```python
from build123d import *

# Parameters (mm, degrees)
F1_DEPTH = 6
F2_R     = 2.5
F3_DEPTH = 50


with BuildPart() as f1:
    # F0 (on Top) → F1 (new body)
    with BuildSketch(Plane.XY):
        Polygon((5, -10), (10, -10), (10, -2), (15, -2), (15, 10), (11, 10), (11, 2), (-11, 2), (-11, 10), (-15, 10), (-15, -2), (-10, -2), (-10, -10), (-5, -10), (-5, -2), (5, -2), align=None)
    extrude(amount=F1_DEPTH)

    # F2 (on face) → F3 (cut)
    with BuildSketch(Plane(origin=(-15, 0, 0), x_dir=(0, -1, 0), z_dir=(-1, 0, 0))):
        with Locations((-6.949849, 3)):
            Circle(F2_R)
        with BuildLine():
            ThreePointArc((-6.949849, 0), (-9.949849, 3), (-6.949849, 6))
            Line((-6.949849, 6), (-10, 6))
            Line((-10, 6), (-10, 0))
            Line((-10, 0), (-6.949849, 0))
        make_face()
        with Locations((6.964043, 3)):
            Circle(F2_R)
        with BuildLine():
            Line((10, 6), (6.964043, 6))
            ThreePointArc((6.964043, 6), (9.085363, 5.12132), (9.964043, 3))
            ThreePointArc((9.964043, 3), (9.085363, 0.87868), (6.964043, 0))
            Line((6.964043, 0), (10, 0))
            Line((10, 0), (10, 6))
        make_face()
    extrude(amount=-F3_DEPTH, mode=Mode.SUBTRACT)


solid = f1.part
```
Build history of the part. All positions in model axes, mm. A direction names the side the tool comes from. Coordinates: 2 decimals unless noted, no trailing zeros. Order: outer loops, then holes, each group sorted by start corner. A loop starts at its lowest first (then second) coordinate and runs counter-clockwise, first axis right, second up. Notation, with made-up numbers: (87, 18.25) -> (127, 18.25) arc R12 ccw to (127, 32.25) -> close; hole circle Ø4 at (81, 49.5). An arc over 180 degrees is marked (long way). Answer in a Markdown table with one row per item. Add a question column.
Q1. Which spindle directions (+Z, -Z, +X, -X, +Y, -Y) get a long thin tool onto all of the face, cutting with end or side? Do faces 4 (the face through (-13, -2, 3)), 5 (the face through (0, 2, 3)), 6 (the face through (12, -2, 3)), 7 (the face through (0, -2, 3)). Say none if no direction does.
Q2. Drop flat-ended pins along their axis: pin 1 (1.5 mm diameter, centred on x = -6, z = 4.5, fed in from -Y); pin 2 (3 mm diameter, centred on y = -6.96, z = 3, fed in from -X); pin 3 (3 mm diameter, centred on x = -9, z = 4, fed in from +Y); pin 4 (1.8 mm diameter, centred on y = -4.5, z = 2.5, fed in from -X). Give the stop position or say it passes through.
Q3. Mould opens along Y. For faces 1 (the face through (12.97, 9.95, 2.93)), 2 (the face through (0, 0, 0)), 3 (the face through (-13.028, 9.447, 3.11)) say: +Y half, -Y half, draft (parallel to the pull), parting line (faces both ways), or undercut.
Q4. Band-saw the part on D-D, the plane z = 4. Give the number of separate pieces and of enclosed holes in the cut face, then the cut area to 3 significant figures.
Q5. Wall check: line 1 along X through (y, z) = (-3.5, 5); line 2 along X through (y, z) = (2.75, 5.5); line 3 along Y through (x, z) = (12.5, 1.25). Give the ranges that are in metal, low to high. Write a range as [from, to].
Q6. Band-saw the part on C-C, the plane y = -8.75. List the corners of the cut face in (x, z), then the cut area to 3 significant figures.
Q7. Band-saw the part on A-A, the plane y = -4. List the corners of the cut face in (x, z), then the cut area to 3 significant figures.
Q8. Band-saw the part on B-B, the plane x = 9.5. List the corners of the cut face in (y, z).
Answers follow:
| question | item | result |
|---|---|---|
| 1 | face 4 | +Z, -Z, -X, -Y |
| 1 | face 5 | +Z, -Z, +Y |
| 1 | face 6 | +Z, -Z, +X, -Y |
| 1 | face 7 | +Z, -Z, -Y |
| 2 | pin 1 | y = -9.87 |
| 2 | pin 2 | through |
| 2 | pin 3 | y = 2 |
| 2 | pin 4 | x = -10 |
| 3 | face 1 | +Y half |
| 3 | face 2 | draft |
| 3 | face 3 | undercut |
| 4 | separate pieces | 5 |
| 4 | enclosed holes | 0 |
| 4 | area | 178 mm^2 |
| 5 | line 1 | [-10, -5], [5, 10] |
| 5 | line 2 | [-15, -11], [11, 15] |
| 5 | line 3 | [-2, 5.16], [8.74, 9.39] |
| 6 | outline | (-10, 0.59) -> (-5, 0.59) -> (-5, 1.25) -> (-10, 1.25) -> close; (-10, 4.75) -> (-5, 4.75) -> (-5, 5.41) -> (-10, 5.41) -> close; (5, 0.59) -> (10, 0.59) -> (10, 1.25) -> (5, 1.25) -> close; (5, 4.75) -> (10, 4.75) -> (10, 5.41) -> (5, 5.41) -> close |
| 6 | area | 13.2 mm^2 |
| 7 | outline | (-10, 0) -> (-5, 0) -> (-5, 6) -> (-10, 6) -> close; (5, 0) -> (10, 0) -> (10, 6) -> (5, 6) -> close |
| 7 | area | 60.0 mm^2 |
| 8 | outline | (-9.96, 3) arc R3 ccw to (-6.96, 0) -> (2, 0) -> (2, 6) -> (-6.96, 6) arc R3 ccw to start; hole circle Ø5 at (-6.96, 3) |
